```python
from build123d import *

# Parameters (mm, degrees)
F0_W     = 60
F0_H     = 128
F1_ANGLE = 10
F3_DEPTH = 60.001
F4_W     = 60
F4_H     = 96
F4_R     = 4
F5_DEPTH = 2
F4_R_2   = 1.5
F6_DEPTH = 8


with BuildPart() as f1:
    # F0 (on Top) → F1 (revolve)
    with BuildSketch(Plane.XY):
        with Locations((-4.03933, 18.915136)):
            Rectangle(F0_W, F0_H)
    revolve(axis=Axis((-4.03933, -45.084864, 0), (1, 0, 0)), revolution_arc=F1_ANGLE)

    # F2 (on face) → F3 (cut, through all)
    with BuildSketch(Plane.YZ.offset(25.96067)):
        with BuildLine():
            Line((80.970529, 22.226967), (82.915136, 0))
            ThreePointArc((82.915136, 0), (82.428058, 11.155935), (80.970529, 22.226967))
        make_face()
    extrude(amount=-F3_DEPTH, mode=Mode.SUBTRACT)

    # F4 (on face) → F5 (cut)
    with BuildSketch(Plane(origin=(0, 0, 0), x_dir=(1, 0, 0), z_dir=(0, 0, -1))):
        with Locations((-4.03933, -34.915136)):
            Rectangle(F4_W, F4_H)
        with Locations((-28.03933, -74.915136)):
            Circle(F4_R, mode=Mode.SUBTRACT)
        with Locations((19.96067, -74.915136)):
            Circle(F4_R, mode=Mode.SUBTRACT)
        with Locations((-28.03933, -10.915136)):
            Circle(F4_R, mode=Mode.SUBTRACT)
        with Locations((19.96067, -10.915136)):
            Circle(F4_R, mode=Mode.SUBTRACT)
    extrude(amount=-F5_DEPTH, mode=Mode.SUBTRACT)

    # F4 (on face) → F6 (cut)
    with BuildSketch(Plane(origin=(0, 0, 0), x_dir=(1, 0, 0), z_dir=(0, 0, -1))):
        with Locations((-28.03933, -10.915136)):
            Circle(F4_R_2)
        with Locations((19.96067, -10.915136)):
            Circle(F4_R_2)
        with Locations((19.96067, -74.915136)):
            Circle(F4_R_2)
        with Locations((-28.03933, -74.915136)):
            Circle(F4_R_2)
    extrude(amount=-F6_DEPTH, mode=Mode.SUBTRACT)


solid = f1.part
```
Geometry check sheet. Reference: the model listing, model coordinates, mm. A direction names the side the tool comes from. Round coordinates to 2 decimals unless told otherwise and drop trailing zeros. Loops run counter-clockwise (first coordinate to the right, second up) from the corner with the lowest first, then second, coordinate; pieces in that order, holes last. Notation, with made-up numbers: (-33.5, -39.75) -> (-19.5, -39.75) arc R17 cw to (-19.5, -35.75) -> close; hole circle Ø6 at (44, 5.25). An arc over 180 degrees is marked (long way). Use a Markdown table: item, result.
(1) Sectioned sample at A-A (x = -17.5). Enter the section's corners in (y, z), then the cut area to 3 significant figures.
Calculated:
| item | result |
|---|---|
| outline | (-45.08, 0) -> (-13.08, 0) -> (-13.08, 2) -> (82.74, 2) -> (80.97, 22.23) -> close |
| area | 1,230 mm² |
(2) Go/stop test with flat-tipped pins: P1, Ø8, axis at x = -15.5, y = 38, coming from the -Z side; P2, Ø5, axis at x = -14, y = -19.5, coming from the +Z side; P3, Ø1.5, axis at x = 2, z = 19.5, coming from the +Y side. Record where each tip stops, or that it passes through.
Calculated:
| item | result |
|---|---|
| P1 | z = 2 |
| P2 | z = 4.95 |
| P3 | y = 81.27 |
(3) Scan lines: probe 1 along Z at (x, y) = (6, -16); probe 2 along Z at (x, y) = (22.5, 62). Record each from-to range of solid material in increasing order.
Calculated:
| item | result |
|---|---|
| probe 1 | 0 to 5.13 |
| probe 2 | 2 to 18.88 |
(4) Sectioned sample at D-D (z = 19.75). Enter the section's corners in (x, y), then the cut area to 3 significant figures.
Calculated:
| item | result |
|---|---|
| outline | (-34.04, 66.92) -> (25.96, 66.92) -> (25.96, 81.19) -> (-34.04, 81.19) -> close |
| area | 856 mm² |
(5) Sectioned sample at B-B (z = 6). Enter the section's corners in (x, y), then the cut area to 3 significant figures.
Calculated:
| item | result |
|---|---|
| outline | (-34.04, -11.06) -> (25.96, -11.06) -> (25.96, 82.39) -> (-34.04, 82.39) -> close; hole circle Ø3 at (-28.04, 10.92); hole circle Ø3 at (-28.04, 74.92); hole circle Ø3 at (19.96, 10.92); hole circle Ø3 at (19.96, 74.92) |
| area | 5,580 mm² |
(6) Mould release check, pull along X, two halves, no side actions. Record for faces 3 (the flat face through (20, 73, 0)), 4 (the cylindrical face through (23.776, 9.714, 0.986)), 5 (the flat face through (25.961, 34, 9)): released by +X, released by -X, zero draft, split by the parting line, or undercut.
Calculated:
| item | result |
|---|---|
| face 3 | zero draft |
| face 4 | undercut |
| face 5 | released by +X |
(7) Sectioned sample at C-C (y = -2). Enter the section's corners in (x, z).
Calculated:
| item | result |
|---|---|
| outline | (-34.04, 2) -> (25.96, 2) -> (25.96, 7.6) -> (-34.04, 7.6) -> close |
(8) Set-up check for faces 1 (the flat face through (20, 9, 0)), 2 (the flat face through (-28, 75, 8)): record each of +Z, -Z, +X, -X, +Y, -Y from which the full face is reachable in a straight line by a thin tool's end or side.
Calculated:
| item | result |
|---|---|
| face 1 | -Z, +X, -X, +Y, -Y |
| face 2 | -Z |
